Autodesk Fusion 360 part; units mm, degrees
sketch "Esquisse1" plane through (0, 0, 0) normal (0, 0, 1) x (1, 0, 0)
  line L0 (0, 0) -> (25, 0) construction
  line L1 (0, 0) -> (0, 1.8)
  line L2 (0, 1.8) -> (4, 1.8)
  line L3 (4, 1.8) -> (4, 5)
  line L4 (4, 5) -> (19, 5)
  line L5 (19, 5) -> (19, 0)
  arc A0 (5.3, 5) -> (17.7, 5) centre (11.5, 15.4559) ccw
  line L6 (0, 0) -> (19, 0)
  line L7 (7.6902, 3.3) -> (16, 3.3) construction
  dimension "d1" = 1.8
  dimension "d2" = 4
  dimension "d3" = 5
  dimension "d4" = 1.3
  dimension "d5" = 1.3
  dimension "d12" = 15
  dimension "d14" = 3.3
revolve "Révolution1" add sketch "Esquisse1" angle 360 about axis through (0, 0, 0) along (1, 0, 0) contours L1 L2 L3 L4 L5 A0 L6
fillet "Congé1" radius 0.5 2 edges at (19, -1.8081, 4.6616) (4, -1.8081, 4.6616)
fillet "Congé2" radius 0.5 1 edges at (0, -0.6509, 1.6782)
Build history of the part. All positions in model axes, mm. A direction names the side the tool comes from. Coordinates: 2 decimals unless noted, no trailing zeros. Order: outer loops, then holes, each group sorted by start corner. A loop starts at its lowest first (then second) coordinate and runs counter-clockwise, first axis right, second up. Notation, with made-up numbers: (20.5, -3.5) -> (26.5, -3.5) arc R5 cw to (26.5, 3.5) -> close; hole circle Ø10 at (83, 0.25). An arc over 180 degrees is marked (long way). Answer in a Markdown table with one row per item. Add a question column.
Q1. Band-saw the part on C-C, the plane x = 11.5. List the corners of the cut face in (y, z).
Q2. Band-saw the part on A-A, the plane y = 0. List the corners of the cut face in (x, z).
Q3. Wall check: line 1 along X through (y, z) = (-1.5, -1.75); line 2 along X through (y, z) = (-4.5, 2); line 3 along X through (y, z) = (-3, -3.75). Give the ranges that are in metal, low to high. Write a range as [from, to].
Q4. Drop flat-ended pins along their axis: pin 1 (3 mm diameter, centred on x = 14.5, z = 1.5, fed in from -Y); pin 2 (3 mm diameter, centred on x = 8, y = -0.5, fed in from +Z); pin 3 (1 mm diameter, centred on x = 15.5, y = -3, fed in from -Z). Give the stop position or say it passes through.
Q5. Which spindle directions (+Z, -Z, +X, -X, +Y, -Y) get a long thin tool onto all of the face, cutting with end or side? Do faces 1 (the face through (19, 0, 0)), 2 (the face through (4, 0, -2)). Say none if no direction does.
Answers follow:
| question | item | result |
|---|---|---|
| 1 | outline | circle Ø6.6 at (0, 0) |
| 2 | outline | (0, -1.3) arc R0.5 ccw to (0.5, -1.8) -> (4, -1.8) -> (4, -4.5) arc R0.5 ccw to (4.5, -5) -> (5.3, -5) arc R12.16 cw to (17.7, -5) -> (18.5, -5) arc R0.5 ccw to (19, -4.5) -> (19, 4.5) arc R0.5 ccw to (18.5, 5) -> (17.7, 5) arc R12.16 cw to (5.3, 5) -> (4.5, 5) arc R0.5 ccw to (4, 4.5) -> (4, 1.8) -> (0.5, 1.8) arc R0.5 ccw to (0, 1.3) -> close |
| 3 | line 1 | [4, 19] |
| 3 | line 2 | [4.24, 5.43], [17.57, 18.76] |
| 3 | line 3 | [4.1, 5.65], [17.35, 18.9] |
| 4 | pin 1 | y = -4.02 |
| 4 | pin 2 | z = 4.36 |
| 4 | pin 3 | z = -3.15 |
| 5 | face 1 | +Z, -Z, +X, +Y, -Y |
| 5 | face 2 | -X |
